from build123d import *

# Parameters (mm, degrees)
F1_DEPTH = 29
F3_DEPTH = 38.001
F5_DEPTH = 18
F6_R     = 5


with BuildPart() as f1:
    # F0 (on Front) → F1 (new body, symmetric)
    with BuildSketch(Plane.XZ):
        with BuildLine():
            Line((0, 9), (0, 0))
            Line((0, 0), (105, 0))
            Line((105, 0), (105, 9))
            Line((105, 9), (116, 9))
            ThreePointArc((116, 9), (114.7027189695, 25.0941347815), (105, 38))
            Line((105, 38), (0, 38))
            ThreePointArc((0, 38), (-9.7027189695, 25.0941347815), (-11, 9))
            Line((-11, 9), (0, 9))
        make_face()
    extrude(amount=F1_DEPTH, both=True)

    # F2 (on face) → F3 (cut, through all)
    with BuildSketch(Plane.XY.offset(38)):
        with BuildLine():
            ThreePointArc((14, 6.5), (7.5, 0), (14, -6.5))
            Line((14, -6.5), (33, -6.5))
            ThreePointArc((33, -6.5), (39.5, 0), (33, 6.5))
            Line((33, 6.5), (14, 6.5))
        make_face()
        with BuildLine():
            ThreePointArc((72, 6.5), (65.5, 0), (72, -6.5))
            Line((72, -6.5), (91, -6.5))
            ThreePointArc((91, -6.5), (97.5, 0), (91, 6.5))
            Line((91, 6.5), (72, 6.5))
        make_face()
    extrude(amount=-F3_DEPTH, mode=Mode.SUBTRACT)

    # F4 (on Front) → F5 (cut, symmetric)
    with BuildSketch(Plane.XZ):
        with BuildLine():
            Line((105, 38), (0, 38))
            ThreePointArc((0, 38), (-5.1316907331, 33.0512170183), (-8.9009712184, 27))
            Line((-8.9009712184, 27), (113.9009712184, 27))
            ThreePointArc((113.9009712184, 27), (110.1316907331, 33.0512170183), (105, 38))
        make_face()
    extrude(amount=F5_DEPTH, both=True, mode=Mode.SUBTRACT)

    # F6
    f6_edges = [f1.edges().sort_by_distance(p)[0] for p in [
        (114.702719, 29, 25.094135),
        (52.5, 29, 38),
        (-9.702719, 29, 25.094135),
        (114.702719, -29, 25.094135),
        (52.5, -29, 38),
        (-9.702719, -29, 25.094135),
    ]]
    fillet(f6_edges, radius=F6_R)


solid = f1.part
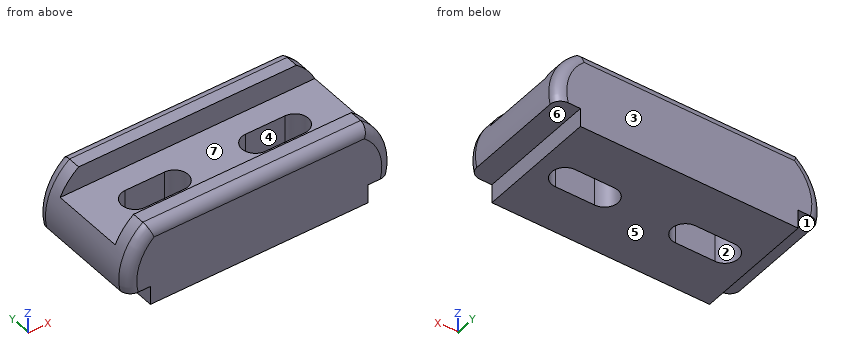
Could you check a few things on this model? Use its own coordinates, in mm. Face numbers are marked on the shaded views. A direction names the side the tool comes from. Give positions to 0.01 mm unless a question says otherwise; leave off trailing zeros. Order: outer loops, then holes, each group sorted by start corner. A loop starts at its lowest first (then second) coordinate and runs counter-clockwise, first axis right, second up.
1. Suppose I cut it at B-B (y = 0). Write out the boundary of the cut face in (x, z).
Answers below:
outline: (-11, 9) - (0, 9) - (0, 0) - (7.5, 0) - (7.5, 27) - (-8.9, 27) arc R29 ccw to start; (39.5, 0) - (65.5, 0) - (65.5, 27) - (39.5, 27) - close; (97.5, 0) - (105, 0) - (105, 9) - (116, 9) arc R29 ccw to (113.9, 27) - (97.5, 27) - close
2. Suppose I cut it at C-C (z = 3). Write out the boundary of the cut face in (x, y), plus the area to 3 significant figures.
Answers below:
outline: (0, -29) - (105, -29) - (105, 29) - (0, 29) - close; hole (14, -6.5) - (33, -6.5) arc R6.5 ccw to (33, 6.5) - (14, 6.5) arc R6.5 ccw to start; hole (72, -6.5) - (91, -6.5) arc R6.5 ccw to (91, 6.5) - (72, 6.5) arc R6.5 ccw to start
area: 5,330 mm2
3. Suppose I cut it at A-A (x = 82). Write out the boundary of the cut face in (y, z).
Answers below:
outline: (-29, 0) - (-6.5, 0) - (-6.5, 27) - (-18, 27) - (-18, 38) - (-24, 38) arc R5 ccw to (-29, 33) - close; (6.5, 0) - (29, 0) - (29, 33) arc R5 ccw to (24, 38) - (18, 38) - (18, 27) - (6.5, 27) - close
4. Suppose I cut it at D-D (x = 3). Write out the boundary of the cut face in (y, z).
Answers below:
outline: (-29, 0) - (29, 0) - (29, 33) arc R5 ccw to (24, 38) - (18, 38) - (18, 27) - (-18, 27) - (-18, 38) - (-24, 38) arc R5 ccw to (-29, 33) - close
5. For pin 1 (8 mm diameter, centred on y = -19.5, z = 9, fed in from -X); pin 2 (18 mm diameter, centred on x = 31.5, y = 3, fed in from +Z); pin 3 (3.5 mm diameter, centred on x = 112.5, y = 13.5, fed in from -Z), each with a flat end and sliding along its axis, tell me the tip position at first contact or that it passes through.
Answers below:
pin 1: stops at x = -11.53
pin 2: stops at z = 27
pin 3: stops at z = 9
6. Thinking about a two-plate mould opening in Y: for the marked faces 1, 2 and 3, which applies, +Y half, -Y half, draft (parallel to the pull), parting line (faces both ways), or undercut?
Answers below:
face 1: draft
face 2: undercut
face 3: +Y half
7. Which directions (+Z, -Z, +X, -X, +Y, -Y) give clear straight access to the entire face, cutting with the end or side of a thin tool? Please do the marked faces 4, 5, 6 and 7.
Answers below:
face 4: +Z, -Z
face 5: -Z, +X, -X, +Y, -Y
face 6: -Z, +X, +Y, -Y
face 7: +Z, +X, -X
8. I need wall thicknesses on L1, parallel to Y at x = 20.5, z = 17; L2, parallel to Y at x = 63, z = 31.5; L3, parallel to Z at x = 72.5, y = -7. Which ranges of each line are inside material? Lowest first, please.
Answers below:
L1: y = -29 to -6.5, 6.5 to 29
L2: y = -29 to -18, 18 to 29
L3: z = 0 to 27
